```python
from build123d import *

# Parameters (mm, degrees)
SKETCH2_W            = 30
SKETCH2_H            = 62
BOSS_EXTRUDE10_DEPTH = 5
SKETCH1_R            = 1
CUT_EXTRUDE5_DEPTH   = 1.5
SKETCH1_14_R         = 1
CUT_EXTRUDE6_DEPTH   = 35.799425283
FILLET1_R            = 15
SKETCH5_W            = 30
SKETCH5_H            = 5
BOSS_EXTRUDE11_DEPTH = 12.5
FILLET2_R            = 15
SKETCH7_R            = 2.5
CUT_EXTRUDE7_DEPTH   = 3
CHAMFER1_SIZE        = 30
CHAMFER1_SIZE_2      = 15
CHAMFER2_SIZE        = 5
CHAMFER2_SIZE_2      = 15
CUT_EXTRUDE8_DEPTH   = 1.5
SKETCH9_R            = 3.95
CUT_EXTRUDE9_DEPTH   = 10


# Some blends are built 0.0001 mm under size
with BuildPart() as part:
    # Sketch2 → Boss-Extrude10 (new body)
    with BuildSketch(Plane.XY):
        Rectangle(SKETCH2_W, SKETCH2_H)
    extrude(amount=BOSS_EXTRUDE10_DEPTH)

    # Sketch1 → Cut-Extrude5 (cut)
    with BuildSketch(Plane.XY):
        with BuildLine():
            ThreePointArc((2.1, -16), (0, -18.1), (-2.1, -16))
            Line((-2.1, -16), (-3.95, 0))
            Line((-3.95, 0), (-2.1, 16))
            ThreePointArc((-2.1, 16), (0, 18.1), (2.1, 16))
            Line((2.1, 16), (3.95, 0))
            Line((3.95, 0), (2.1, -16))
        make_face()
        with Locations((0, -16)):
            Circle(SKETCH1_R, mode=Mode.SUBTRACT)
        with Locations((0, 16)):
            Circle(SKETCH1_R, mode=Mode.SUBTRACT)
    extrude(amount=CUT_EXTRUDE5_DEPTH, mode=Mode.SUBTRACT)

    # Sketch1<14> → Cut-Extrude6 (cut, through all)
    with BuildSketch(Plane.XY):
        with Locations((0, 16)):
            Circle(SKETCH1_14_R)
        with Locations((0, -16)):
            Circle(SKETCH1_14_R)
    extrude(amount=CUT_EXTRUDE6_DEPTH, mode=Mode.SUBTRACT)

    # Fillet1
    fillet1_edges = [part.edges().sort_by_distance(p)[0] for p in [
        (-15, 31, 2.5),
        (15, 31, 2.5),
    ]]
    fillet(fillet1_edges, radius=FILLET1_R - 0.0001)  # a hair under: the kernel refuses the full size

    # Sketch5 → Boss-Extrude11 (add)
    with BuildSketch(Plane(origin=(0, 0, 0), x_dir=(-1, 0, 0), z_dir=(0, 0, -1))):
        with Locations((0, -28.5)):
            Rectangle(SKETCH5_W, SKETCH5_H)
    boss_extrude11 = extrude(amount=BOSS_EXTRUDE11_DEPTH)

    # Mirror1: Boss-Extrude11 across plane
    add(boss_extrude11.mirror(Plane.XY.offset(2.5)))

    # Fillet2
    # the kernel refuses this fillet: 15 mm, written as the material it takes off along each edge
    with BuildSketch(Plane(origin=(15, 64, 17.5), x_dir=(0, 0, -1), z_dir=(0, -1, 0)), Plane(origin=(-15, -121, 17.5), x_dir=(0, 0, -1), z_dir=(0, 1, 0))) as fillet2_piece_1:
        with BuildLine():
            CenterArc((FILLET2_R, -FILLET2_R), FILLET2_R, 90, 90)
            Line((0, -FILLET2_R), (-FILLET2_R * 0.02, -FILLET2_R))
            Line((-FILLET2_R * 0.02, -FILLET2_R), (-FILLET2_R * 0.02, FILLET2_R * 0.02))
            Line((-FILLET2_R * 0.02, FILLET2_R * 0.02), (FILLET2_R, FILLET2_R * 0.02))
            Line((FILLET2_R, FILLET2_R * 0.02), (FILLET2_R, 0))
        make_face()
    extrude(amount=185, mode=Mode.SUBTRACT)
    with BuildSketch(Plane(origin=(-15, -121, -12.5), x_dir=(0, 0, 1), z_dir=(0, 1, 0)), Plane(origin=(15, 64, -12.5), x_dir=(0, 0, 1), z_dir=(0, -1, 0))) as fillet2_piece_2:
        with BuildLine():
            CenterArc((FILLET2_R, FILLET2_R), FILLET2_R, 180, 90)
            Line((0, FILLET2_R), (-FILLET2_R * 0.02, FILLET2_R))
            Line((-FILLET2_R * 0.02, FILLET2_R), (-FILLET2_R * 0.02, -FILLET2_R * 0.02))
            Line((-FILLET2_R * 0.02, -FILLET2_R * 0.02), (FILLET2_R, -FILLET2_R * 0.02))
            Line((FILLET2_R, -FILLET2_R * 0.02), (FILLET2_R, 0))
        make_face()
    extrude(amount=185, mode=Mode.SUBTRACT)

    # Sketch7 → Cut-Extrude7 (cut)
    with BuildSketch(Plane.XZ.offset(31)):
        with Locations(Location((0, 2.5, 0), (0, 0, 270))):
            Circle(SKETCH7_R)
    extrude(amount=-CUT_EXTRUDE7_DEPTH, mode=Mode.SUBTRACT)

    # Chamfer1
    # the kernel refuses this chamfer: 30, 15 mm, written as the material it adds along each edge
    with BuildSketch(Plane(origin=(-92.485065671, -26, 5), x_dir=(0, 0.9998508956747117, -0.017268075123668125), z_dir=(1, 0, 0))) as chamfer1_piece_1_section:
        Polygon((CHAMFER1_SIZE * 0.999850895675, CHAMFER1_SIZE * 0.0172680751237), (-CHAMFER1_SIZE_2 * 0.0172680751237, CHAMFER1_SIZE_2 * 0.999850895675), (0, 0), align=None)
    chamfer1_piece_1 = extrude(amount=184.970131343, mode=Mode.PRIVATE)
    chamfer1_piece_1 = chamfer1_piece_1 & Plane(origin=(0, -14.759423462, 2.5), x_dir=(0, 0, -1), z_dir=(0, -1, 0)) * Cylinder(15, 490, mode=Mode.PRIVATE)
    chamfer1_piece_1 = chamfer1_piece_1 - Plane(origin=(0, -16, 8.704221218), x_dir=(1, 0, 0), z_dir=(0, 0, -1)) * Cylinder(1, 490, mode=Mode.PRIVATE)
    add(chamfer1_piece_1)

    # Chamfer2
    # the kernel refuses this chamfer: 15, 5 mm, written as the material it adds along each edge
    with BuildSketch(Plane(origin=(-53.716114618, -26, 0), x_dir=(0, 0.9940388851139267, 0.10902612017980706), z_dir=(1, 0, 0))) as chamfer2_piece_1_section:
        Polygon((CHAMFER2_SIZE * 0.994038885114, -CHAMFER2_SIZE * 0.10902612018), (-CHAMFER2_SIZE_2 * 0.10902612018, -CHAMFER2_SIZE_2 * 0.994038885114), (0, 0), align=None)
    chamfer2_piece_1 = extrude(amount=107.432229235, mode=Mode.PRIVATE)
    chamfer2_piece_1 = chamfer2_piece_1 & Plane(origin=(0, -24.267585927, 2.5), x_dir=(0, 0, -1), z_dir=(0, -1, 0)) * Cylinder(15, 275, mode=Mode.PRIVATE)
    add(chamfer2_piece_1)

    # Sketch8 → Cut-Extrude8 (cut)
    with BuildSketch(Plane(origin=(0, 0, 1.5), x_dir=(-1, 0, 0), z_dir=(0, 0, -1))):
        with BuildLine():
            Line((-3.3140625, -5.5), (3.3140625, -5.5))
            Line((3.3140625, -5.5), (3.837114391, -0.976307969))
            ThreePointArc((3.837114391, -0.976307969), (3.893369798, 0), (3.837114391, 0.976307969))
            Line((3.837114391, 0.976307969), (3.3140625, 5.5))
            Line((3.3140625, 5.5), (-3.3140625, 5.5))
            Line((-3.3140625, 5.5), (-3.837114391, 0.976307969))
            ThreePointArc((-3.837114391, 0.976307969), (-3.893369798, 0), (-3.837114391, -0.976307969))
            Line((-3.837114391, -0.976307969), (-3.3140625, -5.5))
        make_face()
    extrude(amount=-CUT_EXTRUDE8_DEPTH, mode=Mode.SUBTRACT)

    # Sketch9 → Cut-Extrude9 (cut)
    with BuildSketch(Plane(origin=(0, 0, 3), x_dir=(-1, 0, 0), z_dir=(0, 0, -1))):
        with Locations(Location((0, 0, 0), (0, 0, 13.230259738))):
            Circle(SKETCH9_R)
    extrude(amount=-CUT_EXTRUDE9_DEPTH, mode=Mode.SUBTRACT)


solid = part.part
```
Work out the finished part from the listing and answer in its coordinate system (mm). A direction names the side the tool comes from. Coordinates: 2 decimals unless noted, no trailing zeros. Loops run counter-clockwise (first coordinate to the right, second up) from the corner with the lowest first, then second, coordinate; pieces in that order, holes last. Notation, with made-up numbers: M 44,78 L 68,78 A25 ccw 68,112 Z; hole C 47,29 d2. An arc over 180 degrees is marked long. Use CSV: the item, a comma, the result in double quotes. Start each with the question number.
(1) Given pin 1 Ø2.5 at (x, y) = (0, 16) entering from -Z; pin 2 Ø13.5 at (x, y) = (3.5, 16) entering from +Z; pin 3 Ø0.8 at (x, z) = (1.5, 2.5) entering from +Y; pin 4 Ø5 at (y, z) = (2, 11) entering from +X, each flat-ended and moving along its own axis, determine where each tip first touches the part or whether it passes through.
(2) For faces 1 (the face through (-0.05, -3.95, 5.29)), 2 (the face through (0.1, -4.2, 3)), 3 (the face through (-3.893, -0.014, 2.24)), determine the directions among +Z, -Z, +X, -X, +Y, -Y from which every point of the face is accessible in a straight line to the end or side of a thin tool.
(3) Find section B-B, the plane z = -5. Give the vertices of the cut face in (x, y).
(4) For a pull along X with two mould halves and no side action, classify faces 4 (the face through (0, -31, 6)), 5 (the face through (-10.72, 26.49, 2.54)), 6 (the face through (0, -28, 3)) as +X half, -X half, draft (parallel to the pull), parting line (faces both ways), or undercut.
(5) Find section C-C, the plane x = 5.5. Give the vertices of the cut face in (y, z).
(6) Find section A-A, the plane x = -10. Give the vertices of the cut face in (y, z), then the cut area to 3 significant figures.
(7) Consider line 1 (Y direction, x = 0, z = 4.95); line 2 (Y direction, x = 0, z = 6.35); line 3 (X direction, y = -16, z = 10.75). Determine where each line is inside the solid, lowest interval first.
(8) Find section D-D, the plane y = 25. Give the vertices of the cut face in (x, z).
Recorded:
1,pin 1,"stops at z = 1.5"
1,pin 2,"stops at z = 5"
1,pin 3,"stops at y = 30.96"
1,pin 4,"passes through"
2,face 1,"+Z"
2,face 2,"-Z"
2,face 3,"+Z, -Z"
3,outline,"M -12.99,-31 L 12.99,-31 L 12.99,-22.67 L -12.99,-22.67 Z"
4,face 4,"draft"
4,face 5,"-X half"
4,face 6,"undercut"
5,outline,"M -31,-11.46 L -24.82,-11.46 L -21,0 L 29.96,0 L 29.96,5 L 4,5 L -18.91,16.46 L -31,16.46 Z"
6,outline,"M -31,-8.68 L -23.89,-8.68 L -21,0 L 27.18,0 L 27.18,5 L 4,5 L -13.36,13.68 L -31,13.68 Z"
6,area,"594 mm^2"
7,line 1,"y = -28 to -17, -15 to -3.95, 3.95 to 15, 17 to 31"
7,line 2,"y = -31 to -17, -15 to -3.95"
7,line 3,"x = -12.53 to -1, 1 to 12.53"
8,outline,"M -12,0 L 12,0 L 12,5 L -12,5 Z"
